Could you check a few things on this drawing? It's one solid part, dimensions in mm from its lowest x, y, z. A direction names the side the tool comes from. Coordinates: 2 decimals unless noted, no trailing zeros. Loops run counter-clockwise (first coordinate to the right, second up) from the corner with the lowest first, then second, coordinate; pieces in that order, holes last. Notation, with made-up numbers: (-18, 53.25) -> (21, 53.25) arc R16 cw to (21, 61.25) -> close; hole circle Ø11 at (84, 32.25). An arc over 180 degrees is marked (long way). One line per question, with ' | ' between items.
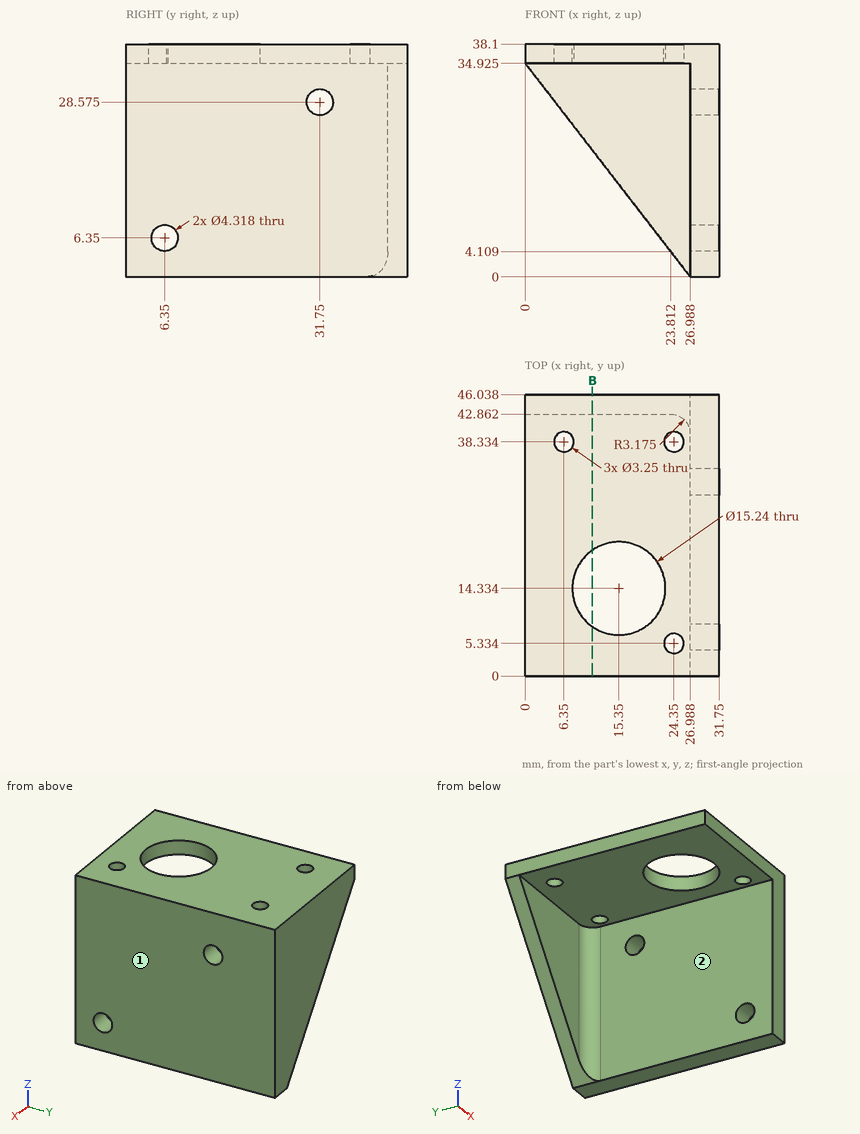
1) If we section it at B-B on x = 11: Please give me the cut outline in (y, z) (1 decimal), and give its area (3 significant figures).
Data:
outline: (0, 34.9) -> (8.1, 34.9) -> (8.1, 38.1) -> (0, 38.1) -> close; (20.6, 34.9) -> (42.9, 34.9) -> (42.9, 20.7) -> (46, 20.7) -> (46, 38.1) -> (20.6, 38.1) -> close | area: 152 mm²
2) I need wall thicknesses on line 1 along Y through (x, z) = (24.35, 37.1); line 2 along Y through (x, z) = (15.35, 36.85) (1 decimal); line 3 along X through (y, z) = (6.5, 22.5). Which ranges of each line are inside material? Lowest first, please. Write a range as from..to.
Data:
line 1: 0..3.71, 6.96..36.71, 39.96..46.04 | line 2: 0..6.7, 22..46 | line 3: 26.99..31.75
3) On a 3-axis mill with a long thin cutter (end or side, diameter ignored), from which of +Z, -Z, +X, -X, +Y, -Y can I reach the whole of each face in a straight line? I mean the marked faces 1 and 2. Say none if no direction works.
Data:
face 1: +Z, -Z, +X, +Y, -Y | face 2: -Z, -X, -Y
4) I'm going to push flat-ended pins straight in: pin 1 Ø2 at (y, z) = (5.5, 13) entering from -X; pin 2 Ø2.5 at (x, y) = (24.35, 5.334) entering from +Z; pin 3 Ø8 at (x, y) = (8.5, 23.5) entering from -Z (1 decimal); pin 4 Ø5 at (x, z) = (22, 21) entering from -Y. Where does each tip first touch, or does it pass through?
Data:
pin 1: x = 26.99 | pin 2: through | pin 3: z = 34.9 | pin 4: y = 42.79
